```python
from build123d import *

# Parameters (mm, degrees)
F0_W     = 81.2292
F0_H     = 56.134
F1_DEPTH = 68.707
F2_W     = 54.3052
F2_H     = 30.1752
F3_DEPTH = 67.056
F4_W     = 7.969416
F4_H     = 6.550535
F5_DEPTH = 165.1


with BuildPart() as f1:
    # F0 (on Front) → F1 (new body, symmetric)
    with BuildSketch(Plane.XZ):
        with Locations((7.321676, 6.277784)):
            Rectangle(F0_W, F0_H)
    extrude(amount=F1_DEPTH, both=True)

    # F2 (on face) → F3 (join, symmetric)
    with BuildSketch(Plane(origin=(0, 68.707, 0), x_dir=(-1, 0, 0), z_dir=(0, 1, 0))):
        with Locations((-8.035632, 5.722342)):
            Rectangle(F2_W, F2_H)
    extrude(amount=F3_DEPTH, both=True)

    # F4 (on face) → F5 (join)
    with BuildSketch(Plane.XY.offset(20.809942)):
        with Locations((-8.885605, 116.388052)):
            Rectangle(F4_W, F4_H)
    extrude(amount=F5_DEPTH)


solid = f1.part
```
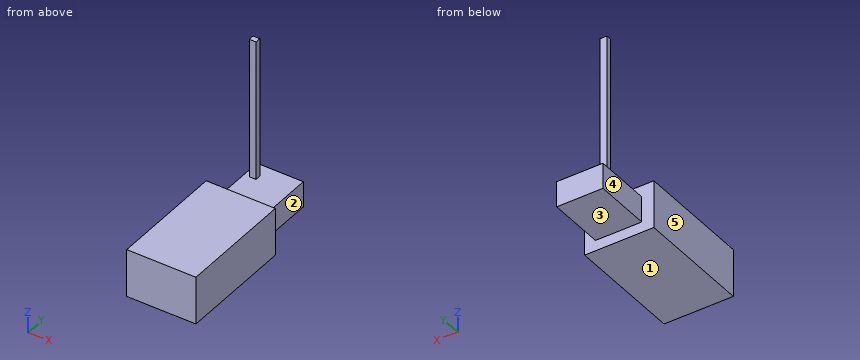
Could you check a few things on this model? Use its own coordinates, in mm. Face numbers are marked on the shaded views. A direction names the side the tool comes from. Give positions to 0.01 mm unless a question says otherwise; leave off trailing zeros. Loops run counter-clockwise (first coordinate to the right, second up) from the corner with the lowest first, then second, coordinate; pieces in that order, holes last. Notation, with made-up numbers: (80.25, 3.5) - (121.25, 3.5) arc R18 ccw to (121.25, 34.5) - close; hole circle Ø3 at (27, 59). An arc over 180 degrees is marked (long way). Answer in a Markdown table with one row per item. Add a question column.
Q1. If we section it at D-D (x = 41): List the corners of the cut face in (y, z) for me, plus the area to 3 significant figures.
Q2. If we section it at C-C (y = 33): List the corners of the cut face in (x, z) for me.
Q3. If we section it at B-B (z = 16): List the corners of the cut face in (x, y) for me.
Q4. Please list where these lines run through material, in increasing order: L1, parallel to X at y = 105.5, z = 7; L2, parallel to Z at x = 6.5, y = 122; L3, parallel to Z at x = -13, y = -14. Write a range as from..to.
Q5. If we section it at A-A (x = 29): List the corners of the cut face in (y, z) for me, plus the area to 3 significant figures.
Q6. For pin 1 (9 mm diameter, centred on y = 118.5, z = 0, fed in from -X); pin 2 (7 mm diameter, centred on y = 115, z = 85.5, fed in from +X); pin 3 (1 mm diameter, centred on x = -13, y = 108, fed in from -Z), each with a flat end and sliding along its axis, tell me the tip position at first contact or that it passes through.
Q7. Which directions (+Z, -Z, +X, -X, +Y, -Y) give clear straight access to the entire face, cutting with the end or side of a thin tool? Please do the marked faces 1, 2, 3, 4 and 5.
The answers:
| question | item | result |
|---|---|---|
| 1 | outline | (-68.71, -21.79) - (68.71, -21.79) - (68.71, 34.34) - (-68.71, 34.34) - close |
| 1 | area | 7,710 mm^2 |
| 2 | outline | (-33.29, -21.79) - (47.94, -21.79) - (47.94, 34.34) - (-33.29, 34.34) - close |
| 3 | outline | (-33.29, -68.71) - (47.94, -68.71) - (47.94, 68.71) - (35.19, 68.71) - (35.19, 135.76) - (-19.12, 135.76) - (-19.12, 68.71) - (-33.29, 68.71) - close |
| 4 | L1 | x = -19.12..35.19 |
| 4 | L2 | z = -9.37..20.81 |
| 4 | L3 | z = -21.79..34.34 |
| 5 | outline | (-68.71, -21.79) - (68.71, -21.79) - (68.71, -9.37) - (135.76, -9.37) - (135.76, 20.81) - (68.71, 20.81) - (68.71, 34.34) - (-68.71, 34.34) - close |
| 5 | area | 9,740 mm^2 |
| 6 | pin 1 | stops at x = -19.12 |
| 6 | pin 2 | stops at x = -4.9 |
| 6 | pin 3 | stops at z = -9.37 |
| 7 | face 1 | -Z, +X, -X, +Y, -Y |
| 7 | face 2 | +Z, -Z, +X, +Y |
| 7 | face 3 | -Z, +X, -X, +Y |
| 7 | face 4 | +Z, -Z, -X, +Y |
| 7 | face 5 | +Z, -Z, -X, +Y, -Y |
